The drawing under review shows one solid part. Ordinate dimensions are in mm from its lowest x, y, z. Round coordinates to 2 decimals unless told otherwise and drop trailing zeros. Order: outer loops, then holes, each group sorted by start corner. A loop starts at its lowest first (then second) coordinate and runs counter-clockwise, first axis right, second up. Notation, with made-up numbers: (-28.5, 6.5) -> (-16.5, 6.5) arc R21 ccw to (-16.5, 38.5) -> close; hole circle Ø5 at (-3, 22). An arc over 180 degrees is marked (long way). Use a Markdown table: item, result. Add a question column.
1) Wall thickness on line 1 along Z through (x, y) = (4.75, 25); line 2 along Y through (x, z) = (3.2, 19); line 3 along Z through (x, y) = (4.3, 10): over which ranges is each line inside the solid? List them lowest first. Write a range as [from, to].
2) Consider section A-A (y = 25). State the section outline as (x, z) points, plus the area to 3 significant figures.
3) Clearance check with flat-ended pins moving along their axes: P1, Ø1.8, axis at x = 4, y = 156, coming from the -Z side; P2, Ø3, axis at x = 2.5, z = 41.5, coming from the -Y side; P3, Ø1.8, axis at x = 2, z = 10, coming from the -Y side; P4, Ø2.5, axis at y = 25, z = 35, coming from the +X side. State where each tip first meets the part, or that it passes through.
4) Consider section D-D (y = 137). State the section outline as (x, z) points.
5) Consider section B-B (x = 3.3). State the section outline as (y, z) points.
6) Consider section C-C (z = 39). State the section outline as (x, y) points.
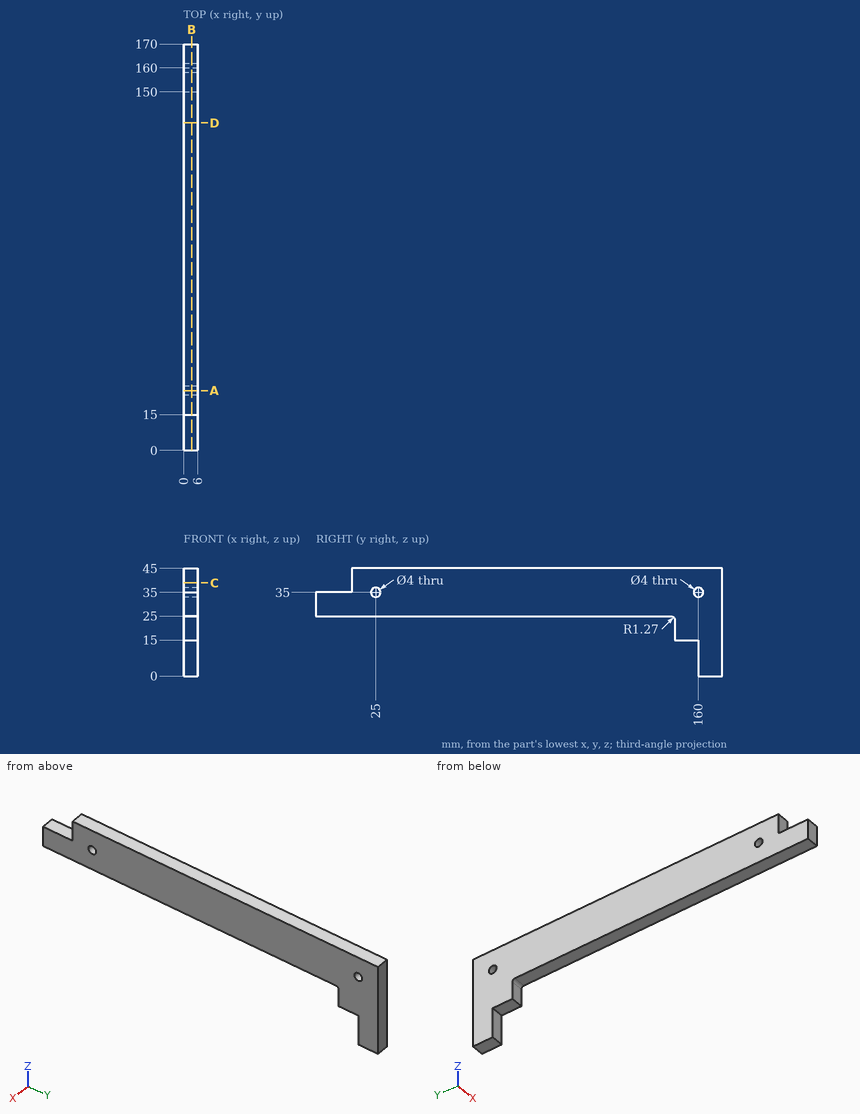
Results list:
| question | item | result |
|---|---|---|
| 1 | line 1 | [25, 33], [37, 45] |
| 1 | line 2 | [150, 170] |
| 1 | line 3 | [25, 35] |
| 2 | outline | (0, 25) -> (6, 25) -> (6, 33) -> (0, 33) -> close; (0, 37) -> (6, 37) -> (6, 45) -> (0, 45) -> close |
| 2 | area | 96.0 mm2 |
| 3 | P1 | z = 15 |
| 3 | P2 | y = 15 |
| 3 | P3 | y = 160 |
| 3 | P4 | through |
| 4 | outline | (0, 25) -> (6, 25) -> (6, 45) -> (0, 45) -> close |
| 5 | outline | (0, 25) -> (148.73, 25) arc R1.27 cw to (150, 23.73) -> (150, 15) -> (160, 15) -> (160, 0) -> (170, 0) -> (170, 45) -> (15, 45) -> (15, 35) -> (0, 35) -> close; hole circle Ø4 at (25, 35); hole circle Ø4 at (160, 35) |
| 6 | outline | (0, 15) -> (6, 15) -> (6, 170) -> (0, 170) -> close |
